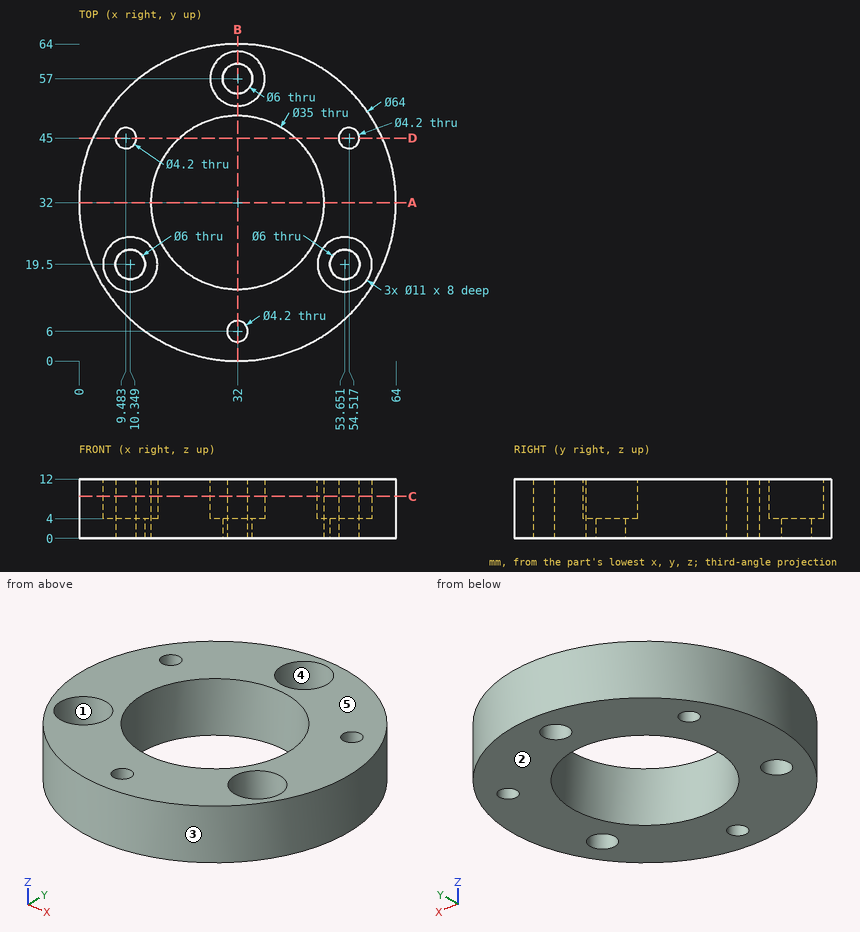
The drawing under review shows one solid part. Ordinate dimensions are in mm from its lowest x, y, z. A direction names the side the tool comes from. Round coordinates to 2 decimals unless told otherwise and drop trailing zeros. Write each loop counter-clockwise with the first axis right and the second up, starting at its lowest first coordinate (ties: lowest second). Pieces come first, ordered by that corner, then holes. Notation, with made-up numbers: (-4.5, 27.5) -> (53.5, 27.5) arc R32 ccw to (53.5, 54.5) -> close; hole circle Ø3 at (5, -27.5). An arc over 180 degrees is marked (long way). One line per question, with ' | ' between items. Start each with the question number.
(1) Mouldability with a two-part tool opening along X and no side actions: class the marked faces 3, 4 and 5 as released by +X, released by -X, zero draft, split by the parting line, or undercut.
(2) For line 1 along Y through (x, z) = (32, 9); line 2 along Y through (x, z) = (32, 2); line 3 along Y through (x, z) = (8, 2) (1 decimal), list the stretches that pass through material, from the lowest coordinate up. Write a range as from..to.
(3) Add section C-C, the plane z = 8.5. Write out the cut boundary in (x, y), plus the area to 3 significant figures.
(4) Add section A-A, the plane y = 32. Write out the cut boundary in (x, z), plus the area to 3 significant figures.
(5) Add section B-B, the plane x = 32. Write out the cut boundary in (y, z).
(6) Add section D-D, the plane y = 45. Write out the cut boundary in (x, z) (1 decimal), plus the area to 3 significant figures.
(7) Insertion check: P1, Ø4, axis at y = 9.5, z = 10, coming from the +X side; P2, Ø5, axis at x = 32, y = 57, coming from the -Z side; P3, Ø5, axis at x = 54.52, y = 45, coming from the -Z side; P4, Ø1.5, axis at x = 37.5, z = 9, coming from the +Y side (1 decimal). Each pin has a flat end and moves straight along its axis. Give the tip position at first contact, or say it passes through.
(8) Tool access review of the marked faces 1 and 2: name each direction out of +Z, -Z, +X, -X, +Y, -Y from which nothing blocks a thin tool from reaching the whole face with its end or side.
Answer list:
1) face 3: split by the parting line | face 4: undercut | face 5: zero draft
2) line 1: 0..3.9, 8.1..14.5, 49.5..51.5, 62.5..64 | line 2: 0..3.9, 8.1..14.5, 49.5..54, 60..64 | line 3: 10.8..17.6, 21.4..43.5, 46.5..53.2
3) outline: circle Ø64 at (32, 32); hole circle Ø11 at (10.35, 19.5); hole circle Ø4.2 at (9.48, 45); hole circle Ø35 at (32, 32); hole circle Ø11 at (32, 57); hole circle Ø4.2 at (32, 6); hole circle Ø11 at (53.65, 19.5); hole circle Ø4.2 at (54.52, 45) | area: 1,930 mm²
4) outline: (0, 0) -> (14.5, 0) -> (14.5, 12) -> (0, 12) -> close; (49.5, 0) -> (64, 0) -> (64, 12) -> (49.5, 12) -> close | area: 348 mm²
5) outline: (0, 0) -> (3.9, 0) -> (3.9, 12) -> (0, 12) -> close; (8.1, 0) -> (14.5, 0) -> (14.5, 12) -> (8.1, 12) -> close; (49.5, 0) -> (54, 0) -> (54, 4) -> (51.5, 4) -> (51.5, 12) -> (49.5, 12) -> close; (60, 0) -> (64, 0) -> (64, 12) -> (62.5, 12) -> (62.5, 4) -> (60, 4) -> close
6) outline: (2.8, 0) -> (7.4, 0) -> (7.4, 12) -> (2.8, 12) -> close; (11.6, 0) -> (20.3, 0) -> (20.3, 12) -> (11.6, 12) -> close; (43.7, 0) -> (52.4, 0) -> (52.4, 12) -> (43.7, 12) -> close; (56.6, 0) -> (61.2, 0) -> (61.2, 12) -> (56.6, 12) -> close | area: 320 mm²
7) P1: x = 56.57 | P2: through | P3: z = 0 | P4: y = 63.6
8) face 1: +Z | face 2: -Z, +X, -X, +Y, -Y
